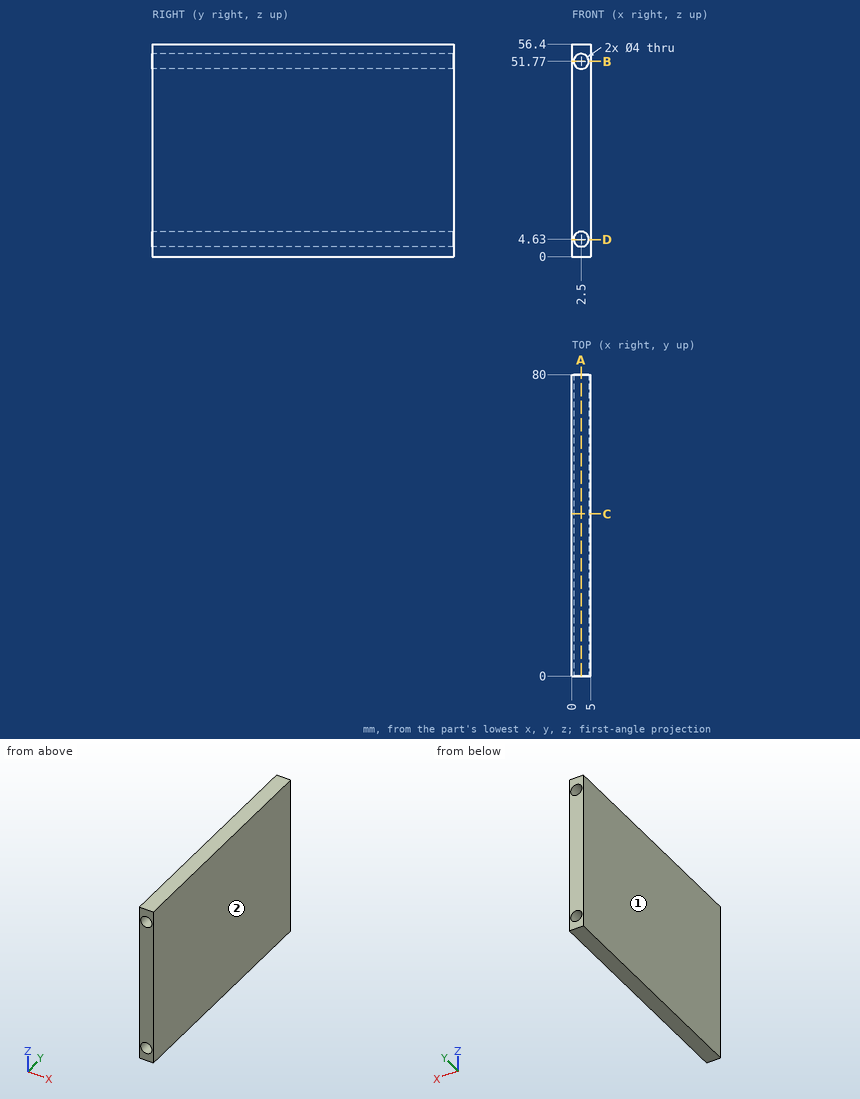
The figure shows three views and two pictorial views of one solid part (mm, origin at its lowest corner). Answer the questions. Coordinates: 2 decimals unless noted, no trailing zeros. Write each loop counter-clockwise with the first axis right and the second up, starting at its lowest first coordinate (ties: lowest second). Pieces come first, ordered by that corner, then holes.
1. For a pull along X with two mould halves and no side action, classify the marked faces 1 and 2 as +X half, -X half, draft (parallel to the pull), parting line (faces both ways), or undercut.
Results list:
face 1: -X half
face 2: +X half
2. Consider line 1 along X through (y, z) = (23, 51.77); line 2 along Z through (x, y) = (2.75, 52); line 3 along Z through (x, y) = (1, 65). Determine where each line is inside the solid, lowest interval first.
Results list:
line 1: x = 0 to 0.5, 4.5 to 5
line 2: z = 0 to 2.65, 6.61 to 49.79, 53.75 to 56.4
line 3: z = 0 to 3.31, 5.95 to 50.45, 53.09 to 56.4
3. The part is cut by section A-A, the plane x = 2.5. Write down the section's boundary in (y, z).
Results list:
outline: (0, 0) - (80, 0) - (80, 2.63) - (0, 2.63) - close; (0, 6.63) - (80, 6.63) - (80, 49.77) - (0, 49.77) - close; (0, 53.77) - (80, 53.77) - (80, 56.4) - (0, 56.4) - close
4. The part is cut by section C-C, the plane y = 43. Write down the section's boundary in (x, z), and give its area (3 significant figures).
Results list:
outline: (0, 0) - (5, 0) - (5, 56.4) - (0, 56.4) - close; hole circle Ø4 at (2.5, 4.63); hole circle Ø4 at (2.5, 51.77)
area: 257 mm2
5. The part is cut by section B-B, the plane z = 51.77. Write down the section's boundary in (x, y).
Results list:
outline: (0, 0) - (0.5, 0) - (0.5, 80) - (0, 80) - close; (4.5, 0) - (5, 0) - (5, 80) - (4.5, 80) - close
6. A flat-ended cylindrical pin translates along its axis: pin 1 (3 mm diameter, centred on x = 2.5, z = 51.77, fed in from -Y). Find the tip coordinate at first contact, or state that the pin passes through.
Results list:
pin 1: passes through
